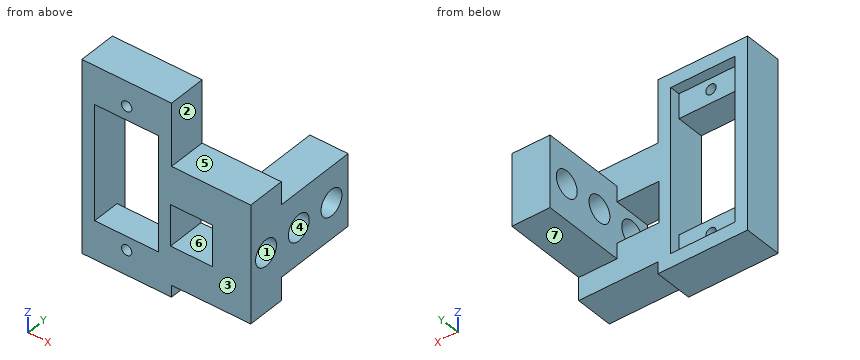
from build123d import *

# Parameters (mm, degrees)
SKETCH4_R           = 1
SKETCH4_W           = 8.2
SKETCH4_H           = 8
SKETCH4_W_2         = 12.5
SKETCH4_H_2         = 22.4
BOSS_EXTRUDE2_DEPTH = 7.46
SKETCH8_W           = 7.46
SKETCH8_H           = 14
BOSS_EXTRUDE4_DEPTH = 16.34
SKETCH9_R           = 2.55
CUT_EXTRUDE2_DEPTH  = 43.142763317
SKETCH12_W          = 12.5
SKETCH12_H          = 32
CUT_EXTRUDE5_DEPTH  = 2


with BuildPart() as part:
    # Sketch4 → Boss-Extrude2 (new body)
    with BuildSketch(Plane(origin=(0, 0, 0), x_dir=(1, 0, 0), z_dir=(0, 1, 0))):
        Polygon((8.75, 11.46), (24.21, 11.46), (24.21, -11.46), (8.75, -11.46), (8.75, -23.65), (-8.75, -23.65), (-8.75, 13.75), (8.75, 13.75), align=None)
        with Locations(Location((0, 8.9, 0), (0, 0, 90))):
            Circle(SKETCH4_R, mode=Mode.SUBTRACT)
        with Locations(Location((0, -18.8, 0), (0, 0, 90))):
            Circle(SKETCH4_R, mode=Mode.SUBTRACT)
        with Locations((12.65, 0)):
            Rectangle(SKETCH4_W, SKETCH4_H, mode=Mode.SUBTRACT)
        with Locations((0, -4.95)):
            Rectangle(SKETCH4_W_2, SKETCH4_H_2, mode=Mode.SUBTRACT)
    extrude(amount=BOSS_EXTRUDE2_DEPTH)

    # Sketch8 → Boss-Extrude4 (add)
    with BuildSketch(Plane(origin=(0, 7.46, 0), x_dir=(1, 0, 0), z_dir=(0, 1, 0))):
        with Locations((20.48, 0)):
            Rectangle(SKETCH8_W, SKETCH8_H)
    extrude(amount=BOSS_EXTRUDE4_DEPTH)

    # Sketch9 → Cut-Extrude2 (cut, through all)
    with BuildSketch(Plane.ZY.offset(-16.75)):
        with Locations((0, 3.73)):
            Circle(SKETCH9_R)
        with Locations((0, 11.73)):
            Circle(SKETCH9_R)
        with Locations((0, 19.73)):
            Circle(SKETCH9_R)
    extrude(amount=-CUT_EXTRUDE2_DEPTH, mode=Mode.SUBTRACT)

    # Sketch12 → Cut-Extrude5 (cut)
    with BuildSketch(Plane(origin=(0, 7.46, 0), x_dir=(1, 0, 0), z_dir=(0, 1, 0))):
        with Locations((0, -4.95)):
            Rectangle(SKETCH12_W, SKETCH12_H)
    extrude(amount=-CUT_EXTRUDE5_DEPTH, mode=Mode.SUBTRACT)


solid = part.part
Source: CAD feature listing. Evaluate the final solid. Frame: model axes, mm. Face numbers are marked on the shaded views. A direction names the side the tool comes from. Give positions to 0.01 mm unless a question says otherwise; leave off trailing zeros. Loops run counter-clockwise (first coordinate to the right, second up) from the corner with the lowest first, then second, coordinate; pieces in that order, holes last. Notation, with made-up numbers: (73, 35.25) -> (104, 35.25) arc R13 cw to (104, 39.25) -> close; hole circle Ø6 at (-19, 75). An arc over 180 degrees is marked (long way). Use a Markdown table: item, result. Add a question column.
1) First-contact query: pin 1 (1.8 mm diameter, centred on x = 0, z = 18.8, fed in from -Y); pin 2 (6 mm diameter, centred on x = 22, y = 18, fed in from -Z); pin 3 (10 mm diameter, centred on x = 15, y = 6, fed in from +Z); pin 4 (8 mm diameter, centred on x = 19, y = 17, fed in from +Z). Flat tips, straight axial feed; report the tip coordinate or a pass-through.
2) Section query D-D, the plane y = 3.73. Return the cut outline in (x, z).
3) Reachability of the marked faces 5, 6 and 7 from +Z, -Z, +X, -X, +Y, -Y: full face, straight path, thin tool, end or side. Return the list, or none.
4) Section query C-C, the plane x = 3. Return the cut outline in (y, z).
5) Line query: line 1 along Y through (x, z) = (19.5, 0); line 2 along X through (y, z) = (2, -1.5); line 3 along X through (y, z) = (12.75, -2.5). Output: solid intervals per line, ascending. Write a range as [from, to].
6) Pull-direction query (Y, two-part tool) for the marked faces 1, 2, 3 and 4; classes: +Y half, -Y half, draft (parallel to the pull), parting line (faces both ways), or undercut.
7) Section query A-A, the plane y = 19.73. Return the cut outline in (x, z).
8) Section query B-B, the plane z = 8. Return the cut outline in (x, y).
Numbers:
| question | item | result |
|---|---|---|
| 1 | pin 1 | passes through |
| 1 | pin 2 | stops at z = -7 |
| 1 | pin 3 | stops at z = 11.46 |
| 1 | pin 4 | stops at z = 7 |
| 2 | outline | (-8.75, -13.75) -> (8.75, -13.75) -> (8.75, -11.46) -> (24.21, -11.46) -> (24.21, -2.55) -> (16.75, -2.55) -> (16.75, -4) -> (8.55, -4) -> (8.55, 4) -> (16.75, 4) -> (16.75, 2.55) -> (24.21, 2.55) -> (24.21, 11.46) -> (8.75, 11.46) -> (8.75, 23.65) -> (-8.75, 23.65) -> close; hole (-6.25, -6.25) -> (6.25, -6.25) -> (6.25, 16.15) -> (-6.25, 16.15) -> close; hole circle Ø2 at (0, -8.9); hole circle Ø2 at (0, 18.8) |
| 3 | face 5 | +Z, +X, +Y, -Y |
| 3 | face 6 | +Y, -Y |
| 3 | face 7 | -Z, +X, -X, +Y |
| 4 | outline | (0, -13.75) -> (7.46, -13.75) -> (7.46, -11.05) -> (5.46, -11.05) -> (5.46, -6.25) -> (0, -6.25) -> close; (0, 16.15) -> (5.46, 16.15) -> (5.46, 20.95) -> (7.46, 20.95) -> (7.46, 23.65) -> (0, 23.65) -> close |
| 5 | line 1 | y = [0, 1.18], [6.28, 9.18], [14.28, 17.18], [22.28, 23.8] |
| 5 | line 2 | x = [-8.75, -6.25], [6.25, 8.55] |
| 5 | line 3 | x = [16.75, 24.21] |
| 6 | face 1 | undercut |
| 6 | face 2 | draft |
| 6 | face 3 | -Y half |
| 6 | face 4 | undercut |
| 7 | outline | (16.75, -7) -> (24.21, -7) -> (24.21, -2.55) -> (16.75, -2.55) -> close; (16.75, 2.55) -> (24.21, 2.55) -> (24.21, 7) -> (16.75, 7) -> close |
| 8 | outline | (-8.75, 0) -> (-6.25, 0) -> (-6.25, 7.46) -> (-8.75, 7.46) -> close; (6.25, 0) -> (24.21, 0) -> (24.21, 7.46) -> (6.25, 7.46) -> close |
